Work out the finished part from the listing and answer in its coordinate system (mm). Face numbers are marked on the shaded views. A direction names the side the tool comes from. Give positions to 0.01 mm unless a question says otherwise; leave off trailing zeros. Write each loop counter-clockwise with the first axis right and the second up, starting at its lowest first coordinate (ties: lowest second). Pieces come first, ordered by that corner, then holes. Notation, with made-up numbers: (37.5, 18) -> (77.5, 18) arc R24 ccw to (77.5, 48) -> close; hole circle Ø4 at (80, -5.5). An arc over 180 degrees is marked (long way). Use a Markdown table: item, result. Add a question column.
Q1. For the marked faces 4, 5 and 6, determine the directions among +Z, -Z, +X, -X, +Y, -Y from which every point of the face is accessible in a straight line to the end or side of a thin tool.
Q2. Section D-D, the plane z = 1.75 is taken. State how many separate pieces and enclosed holes the cut face has, plus the area to 3 significant figures.
Q3. Consider line 1 (X direction, y = 2, z = -3); line 2 (X direction, y = -4, z = -0.5); line 3 (X direction, y = -11.5, z = -3). Determine where each line is inside the solid, lowest interval first.
Q4. Section A-A, the plane x = 0.5 is taken. Give the vertices of the cut face in (y, z).
Q5. For a pull along X with two mould halves and no side action, classify the marked faces 1, 2 and 3 as pulls with the +X half, pulls with the -X half, needs draft (parallel to the pull), parting line crosses it, or undercut.
Q6. Section C-C, the plane x = -7.5 is taken. Give the vertices of the cut face in (y, z).
Q7. Each of these flat-tipped pins is pushed along its axis until it touches: pin 1 Ø2 at (y, z) = (-5, 2) entering from +X; pin 2 Ø1.7 at (x, y) = (20, -8.5) entering from +Z; pin 3 Ø5 at (x, z) = (17.5, -1.5) entering from -Y. Where does it stop, or does it pass through?
Q8. Section B-B, the plane z = -1.5 is taken. Give the vertices of the cut face in (x, y) (3 decimals).
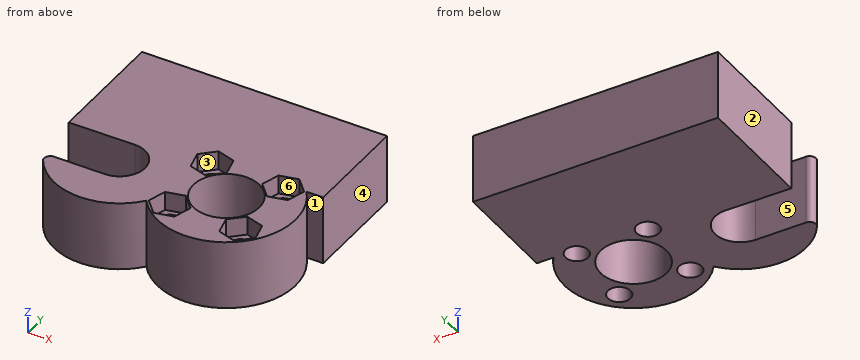
from build123d import *

# Parameters (mm, degrees)
F0_R     = 1.8
F0_R_2   = 5.25
F1_DEPTH = 8
F2_R     = 5.25
F3_DEPTH = 3


with BuildPart() as f1:
    # F0 (on Top) → F1 (new body)
    with BuildSketch(Plane.XY):
        with BuildLine():
            Line((26.1231140105, 19.538577646), (-12.8768859895, 19.538577646))
            Line((-12.8768859895, 19.538577646), (-12.8768859895, 0))
            Line((-12.8768859895, 0), (-2.4018859895, 0.088577646))
            ThreePointArc((-2.4018859895, 0.088577646), (1.6481140105, -3.961422354), (-2.4018859895, -8.011422354))
            Line((-2.4018859895, -8.011422354), (-10.4189381286, -8.011422354))
            ThreePointArc((-10.4189381286, -8.011422354), (-11.2944327118, -8.5281944214), (-11.2650650034, -9.5444038843))
            ThreePointArc((-11.2650650034, -9.5444038843), (-3.0003647918, -14.4193116307), (5.7665147457, -10.5190785227))
            ThreePointArc((5.7665147457, -10.5190785227), (21.1269767102, -12.8143287608), (23.4722336851, 2.538577646))
            Line((23.4722336851, 2.538577646), (26.1231140105, 2.538577646))
            Line((26.1231140105, 2.538577646), (26.1231140105, 19.538577646))
        make_face()
        with Locations((8.941259761, -9.6182766035)):
            Circle(F0_R, mode=Mode.SUBTRACT)
        with Locations((20.2549682599, -9.6182766035)):
            Circle(F0_R, mode=Mode.SUBTRACT)
        with Locations((14.5981140105, -3.961422354)):
            Circle(F0_R_2, mode=Mode.SUBTRACT)
        with Locations((8.941259761, 1.6954318955)):
            Circle(F0_R, mode=Mode.SUBTRACT)
        with Locations((20.2549682599, 1.6954318955)):
            Circle(F0_R, mode=Mode.SUBTRACT)
    extrude(amount=-F1_DEPTH)

    # F2 (on face) → F3 (join)
    with BuildSketch(Plane.XY):
        with BuildLine():
            Line((23.4722336851, 2.538577646), (26.1231140105, 2.538577646))
            Line((26.1231140105, 2.538577646), (26.1231140105, 19.538577646))
            Line((26.1231140105, 19.538577646), (-12.8768859895, 19.538577646))
            Line((-12.8768859895, 19.538577646), (-12.8768859895, 0))
            Line((-12.8768859895, 0), (-2.4018859895, 0.088577646))
            ThreePointArc((-2.4018859895, 0.088577646), (1.6481140105, -3.961422354), (-2.4018859895, -8.011422354))
            Line((-2.4018859895, -8.011422354), (-10.4189381286, -8.011422354))
            ThreePointArc((-10.4189381286, -8.011422354), (-11.2944327118, -8.5281944214), (-11.2650650034, -9.5444038843))
            ThreePointArc((-11.2650650034, -9.5444038843), (-3.0003647918, -14.4193116307), (5.7665147457, -10.5190785227))
            ThreePointArc((5.7665147457, -10.5190785227), (21.1269767102, -12.8143287608), (23.4722336851, 2.538577646))
        make_face()
        Polygon((10.9981298784, -11.8021459494), (8.0784084876, -12.4915130504), (6.0215383702, -10.3076437046), (6.8843896435, -7.4344072576), (9.8041110343, -6.7450401565), (11.8609811518, -8.9289095024), align=None, mode=Mode.SUBTRACT)
        Polygon((19.5656011589, -6.6985552127), (22.4388376058, -7.561406486), (23.1282047069, -10.4811278768), (20.944335361, -12.5379979943), (18.0710989141, -11.6751467209), (17.381731813, -8.7554253301), align=None, mode=Mode.SUBTRACT)
        with Locations((14.5981140105, -3.961422354)):
            Circle(F2_R, mode=Mode.SUBTRACT)
        Polygon((6.7573904151, -0.361438222), (6.068023314, 2.5582831689), (8.2518926599, 4.6151532863), (11.1251291068, 3.752302013), (11.8144962079, 0.8325806222), (9.630626862, -1.2242894953), align=None, mode=Mode.SUBTRACT)
        Polygon((18.1980981425, 3.8793012414), (21.1178195333, 4.5686683425), (23.1746896508, 2.3847989966), (22.3118383774, -0.4884374504), (19.3921169866, -1.1778045514), (17.3352468691, 1.0060647944), align=None, mode=Mode.SUBTRACT)
    extrude(amount=F3_DEPTH)


solid = f1.part
Result set:
| question | item | result |
|---|---|---|
| 1 | face 4 | +Z, -Z, +X, +Y, -Y |
| 1 | face 5 | +Z, -Z, -X |
| 1 | face 6 | +Z |
| 2 | separate pieces | 1 |
| 2 | enclosed holes | 5 |
| 2 | area | 961 mm2 |
| 3 | line 1 | x = -12.88 to 7.17, 10.72 to 18.48, 22.03 to 23.84 |
| 3 | line 2 | x = 1.65 to 9.35, 19.85 to 25.6 |
| 3 | line 3 | x = -9.67 to 4.87, 6.59 to 22.61 |
| 4 | outline | (-14.03, -8) -> (-6.79, -8) -> (-6.79, 3) -> (-14.03, 3) -> close; (-1.14, -8) -> (19.54, -8) -> (19.54, 3) -> (-1.14, 3) -> close |
| 5 | face 1 | needs draft |
| 5 | face 2 | pulls with the -X half |
| 5 | face 3 | undercut |
| 6 | outline | (-13.11, -8) -> (-8.01, -8) -> (-8.01, 3) -> (-13.11, 3) -> close; (0.05, -8) -> (19.54, -8) -> (19.54, 3) -> (0.05, 3) -> close |
| 7 | pin 1 | stops at x = 25.6 |
| 7 | pin 2 | stops at z = 0 |
| 7 | pin 3 | stops at y = -14.95 |
| 8 | outline | (-12.877, 0) -> (-2.402, 0.089) arc R4.05 cw to (-2.402, -8.011) -> (-10.419, -8.011) arc R1 ccw to (-11.265, -9.544) arc R10.475 ccw to (5.767, -10.519) arc R11 ccw to (23.472, 2.539) -> (26.123, 2.539) -> (26.123, 19.539) -> (-12.877, 19.539) -> close; hole circle Ø3.6 at (8.941, -9.618); hole circle Ø3.6 at (8.941, 1.695); hole circle Ø10.5 at (14.598, -3.961); hole circle Ø3.6 at (20.255, -9.618); hole circle Ø3.6 at (20.255, 1.695) |
